Design review of the part built by this model. Coordinates are the model's own, in mm. Face numbers are marked on the shaded views. Give positions to 0.01 mm unless a question says otherwise; leave off trailing zeros. Write each loop counter-clockwise with the first axis right and the second up, starting at its lowest first coordinate (ties: lowest second). Pieces come first, ordered by that corner, then holes.
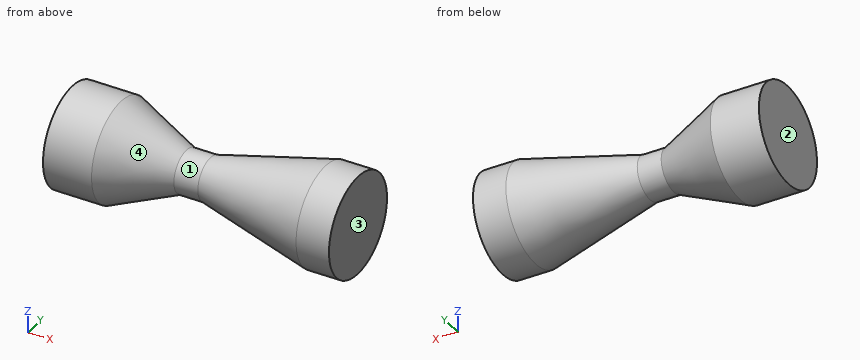
```python
from build123d import *

# Parameters (mm, degrees)
FILLET1_R           = 10
SKETCH2_R           = 35
BOSS_EXTRUDE1_DEPTH = 2
SKETCH3_R           = 34.94624
BOSS_EXTRUDE2_DEPTH = 2


with BuildPart() as part:
    # Sketch1 → Revolve-Thin1 (revolve)
    with BuildSketch(Plane.XY):
        Polygon((-56.494883, 25), (-26.725314, 25), (19.100443, 5), (39.100443, 5), (119.100443, 24.94624), (138.82137, 24.94624), (138.82137, 34.94624), (117.872597, 34.94624), (37.872597, 15), (21.187564, 15), (-24.638193, 35), (-56.494883, 35), align=None)
    revolve(axis=Axis((-43.02316, 0, 0), (1, 0, 0)))

    # Fillet1
    fillet1_edges = [part.edges().sort_by_distance(p)[0] for p in [
        (19.100443, -5, 0),
        (39.100443, -5, 0),
    ]]
    fillet(fillet1_edges, radius=FILLET1_R)

    # Sketch2 → Boss-Extrude1 (add)
    with BuildSketch(Plane.ZY.offset(56.494883)):
        Circle(SKETCH2_R)
    extrude(amount=BOSS_EXTRUDE1_DEPTH)

    # Sketch3 → Boss-Extrude2 (add)
    with BuildSketch(Plane(origin=(138.82137, 0, 0), x_dir=(0, 0, -1), z_dir=(1, 0, 0))):
        Circle(SKETCH3_R)
    extrude(amount=BOSS_EXTRUDE2_DEPTH)


solid = part.part
```
(1) Consider section B-B, the plane z = -9.5. Give the number of separate pieces and of enclosed holes in the cut face, then the cut area to 3 significant figures.
Resolved:
separate pieces: 1
enclosed holes: 2
area: 4,990 mm2
(2) Mouldability with a two-part tool opening along X and no side actions: class the marked faces 1, 2, 3 and 4 as pulls with the +X half, pulls with the -X half, needs draft (parallel to the pull), parting line crosses it, or undercut.
Resolved:
face 1: undercut
face 2: pulls with the -X half
face 3: pulls with the +X half
face 4: undercut
(3) Consider section A-A, the plane x = 111.5. Give the boundary of the cut face in (y, z).
Resolved:
outline: circle Ø66.71 at (0, 0); hole circle Ø46.1 at (0, 0)
(4) Consider section C-C, the plane x = 74. Give the boundary of the cut face in (y, z).
Resolved:
outline: circle Ø48.02 at (0, 0); hole circle Ø27.4 at (0, 0)
(5) To check wall thickness, follow L1, parallel to Z at x = 26.75, y = 0; L2, parallel to Z at x = -36.75, y = 0; L3, parallel to Y at x = -31.5, z = -8.5. State the ranges of each line that lie inside material, in increasing order.
Resolved:
L1: z = -15 to -5, 5 to 15
L2: z = -35 to -25, 25 to 35
L3: y = -33.95 to -23.51, 23.51 to 33.95
(6) Clearance check with flat-ended pins moving along their axes: P1, Ø2, axis at x = -35.5, z = 24.5, coming from the -Y side; P2, Ø6, axis at x = 34.5, z = 11, coming from the +Y side; P3, Ø10, axis at x = 74, z = 2.5, coming from the -Y side. State where each tip first meets the part, or that it passes through.
Resolved:
P1: stops at y = -25.94
P2: stops at y = 12.69
P3: stops at y = -25.18
